```python
from build123d import *

# Parameters (mm, degrees)
F0_R      = 13
F1_DEPTH  = 25
F2_R      = 13
F3_DEPTH  = 3
F4_R      = 2.5
F5_DEPTH  = 25
F0_R_2    = 3
F6_DEPTH  = 30
F8_DEPTH  = 25
F9_DEPTH  = 3.5
F10_DEPTH = 30
F11_R     = 5


# Not quite as in the source:
# - a feature names something its author has since deleted; it is built from what else it names


with BuildPart() as f1:
    # F0 (on Top) → F1 (new body)
    with BuildSketch(Plane.XY):
        with BuildLine():
            Line((-44.2576195002, 24.5322410017), (-44.2576195002, -25.4677589983))
            Line((-44.2576195002, -25.4677589983), (-40.7576195002, -25.4677589983))
            Line((-40.7576195002, -25.4677589983), (-40.7576195002, 34.0321085225))
            Line((-40.7576195002, 34.0321085225), (26.7423804998, 34.0321085225))
            Line((26.7423804998, 34.0321085225), (26.7423804998, 19.5322410017))
            ThreePointArc((26.7423804998, 19.5322410017), (57.445862821, 6.7799260387), (44.8114401571, 37.5321085225))
            Line((44.8114401571, 37.5321085225), (44.6733208426, 37.5321085225))
            Line((44.6733208426, 37.5321085225), (-44.2576195002, 37.5321085225))
            Line((-44.2576195002, 37.5321085225), (-44.2576195002, 24.5322410017))
        make_face()
        with Locations((44.7423804998, 19.5322410017)):
            Circle(F0_R, mode=Mode.SUBTRACT)
    extrude(amount=F1_DEPTH)

    # F2 (on face) → F3 (join)
    with BuildSketch(Plane.XY.offset(25)):
        with BuildLine():
            ThreePointArc((26.7423804998, 19.5322410017), (29.5038185973, 9.9517279079), (36.9408506267, 3.3107696863))
            ThreePointArc((36.9408506267, 3.3107696863), (62.2844095115, 15.4977375434), (44.8114401571, 37.5321085225))
            Line((44.8114401571, 37.5321085225), (-44.2576195002, 37.5321085225))
            Line((-44.2576195002, 37.5321085225), (-44.2576195002, -25.4677589983))
            Line((-44.2576195002, -25.4677589983), (-40.7576195002, -25.4677589983))
            Line((-40.7576195002, -25.4677589983), (-40.7576195002, -15.0916781276))
            Line((-40.7576195002, -15.0916781276), (-40.7576195002, 34.0321085225))
            Line((-40.7576195002, 34.0321085225), (26.7423804998, 34.0321085225))
            Line((26.7423804998, 34.0321085225), (26.7423804998, 19.5322410017))
        make_face()
        with Locations((44.7423804998, 19.5322410017)):
            Circle(F2_R, mode=Mode.SUBTRACT)
    extrude(amount=-F3_DEPTH)

    # F4 (on face) → F5 (cut)
    with BuildSketch(Plane(origin=(-44.2576195002, 0, 0), x_dir=(0, -1, 0), z_dir=(-1, 0, 0))):
        with Locations((12.9677589983, 12.5)):
            Circle(F4_R)
    extrude(amount=-F5_DEPTH, mode=Mode.SUBTRACT)

    # F0 (on Top) → F6 (cut)
    with BuildSketch(Plane.XY):
        with Locations((44.7423804998, 19.5322410017)):
            Circle(F0_R_2)
    extrude(amount=F6_DEPTH, mode=Mode.SUBTRACT)

    # F4 (on face) → F8 (cut)
    with BuildSketch(Plane(origin=(-44.2576195002, 0, 0), x_dir=(0, -1, 0), z_dir=(-1, 0, 0))):
        with Locations((-22.0322410017, 12.5)):
            Circle(F4_R)
    extrude(amount=-F8_DEPTH, mode=Mode.SUBTRACT)

    # F2 (on face) → F9 (join)
    with BuildSketch(Plane.XY.offset(25)):
        with BuildLine():
            Line((18.9116307646, 10.5619383976), (36.9408506267, 3.3107696863))
            ThreePointArc((36.9408506267, 3.3107696863), (29.5038185973, 9.9517279079), (26.7423804998, 19.5322410017))
            Line((26.7423804998, 19.5322410017), (26.7423804998, 34.0321085225))
            Line((26.7423804998, 34.0321085225), (-40.7576195002, 34.0321085225))
            Line((-40.7576195002, 34.0321085225), (-40.7576195002, -15.0916781276))
            Line((-40.7576195002, -15.0916781276), (-14.5708816946, 10.5619383976))
            Line((-14.5708816946, 10.5619383976), (18.9116307646, 10.5619383976))
        make_face()
        with Locations((44.7423804998, 19.5322410017)):
            Circle(F2_R)
    extrude(amount=-F9_DEPTH)

    # F0 (on Top) → F10 (cut)
    with BuildSketch(Plane.XY):
        with Locations((44.7423804998, 19.5322410017)):
            Circle(F0_R_2)
    extrude(amount=F10_DEPTH, mode=Mode.SUBTRACT)

    # F11
    f11_edges = [f1.edges().sort_by_distance(p)[0] for p in [
        (26.74238, 34.032109, 10.75),
        (26.74238, 26.782175, 21.5),
        (-7.00762, 34.032109, 21.5),
        (-40.75762, 34.032109, 10.75),
        (-40.75762, 9.470215, 21.5),
    ]]
    fillet(f11_edges, radius=F11_R)


with BuildPart() as f13_1:
    # F13: instance of F1
    add(f1.part.mirror(Plane.XY.offset(50)))


solid = f13_1.part
```
Design review of the part built by this model. Coordinates are the model's own, in mm. A direction names the side the tool comes from. Round coordinates to 2 decimals unless told otherwise and drop trailing zeros. Order: outer loops, then holes, each group sorted by start corner. A loop starts at its lowest first (then second) coordinate and runs counter-clockwise, first axis right, second up. Notation, with made-up numbers: (3, 35.5) - (62, 35.5) arc R30 cw to (62, 61.5) - close; hole circle Ø6 at (18.25, 80). An arc over 180 degrees is marked (long way). Return JSON: item names as keys, results as strings.
Q1. Consider section A-A on z = 87.5. Write out the cut boundary in (x, y).
Computed values:
{"outline": "(-44.26, -25.47) - (-40.76, -25.47) - (-40.76, -15.47) - (-44.26, -15.47) - close; (-44.26, -10.47) - (-40.76, -10.47) - (-40.76, 19.53) - (-44.26, 19.53) - close; (-44.26, 24.53) - (-40.76, 24.53) - (-40.76, 29.03) arc R5 cw to (-35.76, 34.03) - (21.74, 34.03) arc R5 cw to (26.74, 29.03) - (26.74, 19.53) arc R18 ccw (long way) to (44.81, 37.53) - (-44.26, 37.53) - close; hole circle Ø26 at (44.74, 19.53)"}
Q2. The part is to be moulded in two halves that separate along Z. For faces 1 (the flat face through (45, 23, 78.5)), 2 (the cylindrical face through (-43, -13, 85)), 3 (the flat face through (-44.258, 6, 88)), say which applies: pulls with the +Z half, pulls with the -Z half, needs draft (parallel to the pull), parting line crosses it, or undercut.
Computed values:
{"face 1": "pulls with the +Z half", "face 2": "undercut", "face 3": "needs draft"}
Q3. Consider section C-C on y = -14. Write out the cut boundary in (x, z).
Computed values:
{"outline": "(-44.26, 75) - (-39.64, 75) - (-39.64, 80.35) arc R5 cw to (-40.76, 83.5) - (-40.76, 85.22) - (-44.26, 85.22) - close; (-44.26, 89.78) - (-40.76, 89.78) - (-40.76, 100) - (-44.26, 100) - close"}
Q4. Machinability: for faces 4 (the cylindrical face through (-39.254, 6.661, 79.926)), 5 (the flat face through (2, 10.562, 77)), 6 (the cylindrical face through (56.75, 14.55, 89.4)), which of the approach directions +Z, -Z, +X, -X, +Y, -Y give a long, thin tool a straight path to every point of the face, cutting with its end or side? Answer none if there is none.
Computed values:
{"face 4": "+Z, -Y", "face 5": "+Z, -Z, -Y", "face 6": "+Z"}
Q5. For pin 1 Ø4 at (x, z) = (29.5, 92.5) entering from -Y; pin 2 Ø8 at (x, z) = (-0.5, 90.5) entering from -Y; pin 3 Ø3 at (x, z) = (43, 82.5) entering from -Y; pin 4 Ø5.5 at (x, y) = (44.74, 19.53) entering from +Z, all flat-tipped, find the tip position at first contact; note any pin that passes through.
Computed values:
{"pin 1": "stops at y = 7.34", "pin 2": "stops at y = 34.03", "pin 3": "stops at y = 1.53", "pin 4": "passes through"}
Q6. Consider section D-D on z = 77. Write out the cut boundary in (x, y), plus the area to 3 significant figures.
Computed values:
{"outline": "(-44.26, -25.47) - (-40.76, -25.47) - (-40.76, -15.09) - (-14.57, 10.56) - (18.91, 10.56) - (36.94, 3.31) arc R18 ccw (long way) to (44.81, 37.53) - (-44.26, 37.53) - close; hole circle Ø6 at (44.74, 19.53)", "area": "3,470 mm2"}
Q7. Wall thickness on L1, parallel to Y at x = -43.25, z = 87.5; L2, parallel to Y at x = 5, z = 93.5; L3, parallel to Z at x = 14, y = 13.5: over which ranges is each line inside the solid? List them lowest first. Write a range as [from, to].
Computed values:
{"L1": "y = [-25.47, -15.47], [-10.47, 19.53], [24.53, 37.53]", "L2": "y = [34.03, 37.53]", "L3": "z = [75, 78.5]"}
Q8. Consider section B-B on x = 46. Write out the cut boundary in (y, z), plus the area to 3 significant figures.
Computed values:
{"outline": "(1.58, 75) - (16.81, 75) - (16.81, 78.5) - (6.59, 78.5) - (6.59, 100) - (1.58, 100) - close; (22.26, 75) - (37.49, 75) - (37.49, 100) - (32.47, 100) - (32.47, 78.5) - (22.26, 78.5) - close", "area": "322 mm2"}
